from build123d import *

# Parameters (mm, degrees)
SKETCH1_R           = 2.887093213
BOSS_EXTRUDE1_DEPTH = 2
SKETCH1_4_R         = 2.887093213
SKETCH1_4_R_2       = 1.270321014
BOSS_EXTRUDE2_DEPTH = 1
SKETCH1_6_R         = 1.616772199
BOSS_EXTRUDE5_DEPTH = 5.2
SKETCH3_R           = 5.75
SKETCH3_R_2         = 2.5
SKETCH3_R_3         = 1.1
BOSS_EXTRUDE6_DEPTH = 2.5


with BuildPart() as part:
    # Sketch1 → Boss-Extrude1 (new body)
    with BuildSketch(Plane(origin=(0, 0, 0), x_dir=(1, 0, 0), z_dir=(0, 1, 0))):
        with BuildLine():
            ThreePointArc((45.240075768, -14.546907598), (42.468466284, -11.775298114), (39.6968568, -14.546907598))
            Line((39.6968568, -14.546907598), (35.935854194, -35.366456871))
            ThreePointArc((35.935854194, -35.366456871), (42.66543851, -43.184357012), (48.924361083, -34.984798737))
            Line((48.924361083, -34.984798737), (45.240075768, -14.546907598))
        make_face()
        with Locations(Location((42.470401728, -36.546907513, 0), (0, 0, 270))):
            Circle(SKETCH1_R, mode=Mode.SUBTRACT)
    extrude(amount=BOSS_EXTRUDE1_DEPTH)

    # Sketch1_4 → Boss-Extrude2 (add)
    with BuildSketch(Plane(origin=(0, 0, 0), x_dir=(1, 0, 0), z_dir=(0, 1, 0))):
        with Locations(Location((42.470401728, -36.546907513, 0), (0, 0, 270))):
            Circle(SKETCH1_4_R)
        with Locations(Location((42.470401728, -36.546907513, 0), (0, 0, 270))):
            Circle(SKETCH1_4_R_2, mode=Mode.SUBTRACT)
    extrude(amount=BOSS_EXTRUDE2_DEPTH)

    # Sketch1_6 → Boss-Extrude5 (add)
    with BuildSketch(Plane(origin=(0, 0, 0), x_dir=(1, 0, 0), z_dir=(0, 1, 0))):
        with Locations(Location((42.468466284, -14.546907598, 0), (0, 0, 270))):
            Circle(SKETCH1_6_R)
    extrude(amount=-BOSS_EXTRUDE5_DEPTH)

    # Sketch3 → Boss-Extrude6 (add)
    # profile 1 of 2: a face of its own
    with BuildSketch(Plane.XZ):
        with Locations(Location((42.470401728, 36.546907513, 0), (0, 0, 90))):
            Circle(SKETCH3_R)
        with Locations(Location((42.470401728, 36.546907513, 0), (0, 0, 270))):
            Circle(SKETCH3_R_2, mode=Mode.SUBTRACT)
    # profile 2 of 2: a face of its own
    with BuildSketch(Plane.XZ):
        with Locations((42.470401728, 36.546907513)):
            Circle(SKETCH3_R_3)
    extrude(amount=BOSS_EXTRUDE6_DEPTH)


with BuildPart() as boss_extrude6_kept_piece:
    # of the separate pieces the step leaves, the one the design keeps (boss_extrude6_pieces_kept)
    add(part.part.solids().sort_by_distance((48.924361083, 0, 34.984798737))[0])


solid = boss_extrude6_kept_piece.part
Geometry: final body of the model. Coordinates: model frame, mm. A direction names the side the tool comes from. Coordinates: 2 decimals unless noted, no trailing zeros. Loops run counter-clockwise (first coordinate to the right, second up) from the corner with the lowest first, then second, coordinate; pieces in that order, holes last. Notation, with made-up numbers: (65.5, -4) - (84.5, -4) arc R26 cw to (84.5, 21) - close; hole circle Ø10 at (56.5, 45.25). An arc over 180 degrees is marked (long way). Put each result on its own line as item: value. Start each with the question number.
Q1. Set-up query: faces 4 (the cylindrical face through (42.85, 0.49, 37.76)), 5 (the cylindrical face through (40.89, -2.56, 14.2)), 6 (the cylindrical face through (42.597, 1.493, 33.663)), 7 (the flat face through (44, -2.5, 39)). Return all of +Z, -Z, +X, -X, +Y, -Y with unobstructed straight access to the full face (end or side cutting, diameter ignored); none if empty.
Q2. Pull-direction query (Z, two-part tool) for faces 1 (the flat face through (42, -5.2, 15)), 2 (the flat face through (43, 0, 27)), 3 (the flat face through (37.843, 0.986, 24.811)); classes: released by +Z, released by -Z, zero draft, split by the parting line, or undercut.
Q3. Cut plane C-C, the plane z = 23. Return loops of the section in (x, y), and give its area (3 significant figures).
Q4. Pin query (flat end, axial travel): pin 1 Ø4 at (x, z) = (42, 36) entering from -Y; pin 2 Ø5 at (x, z) = (39.5, 17.5) entering from -Y; pin 3 Ø3 at (y, z) = (0.5, 25) entering from -X; pin 4 Ø4 at (y, z) = (-3.5, 28) entering from -X. Return the tip coordinate at first contact, or that it passes through.
Q5. Line query: line 1 (Z direction, x = 42.5, y = 0.5); line 2 (Z direction, x = 42.25, y = -0.5); line 3 (Y direction, x = 48, z = 40). Output: solid intervals per line, ascending.
Q6. Cut plane A-A, the plane x = 46.75. Return loops of the section in (y, z).
Q7. Cut plane B-B, the plane y = -1.25. Return loops of the section in (x, z).
Q8. Cut plane D-D, the plane y = 1.5. Return loops of the section in (x, z), and give its area (3 significant figures).
Filled sheet:
1. face 4: +Y, -Y
1. face 5: -Y
1. face 6: +Y
1. face 7: +Z, +X, -X, -Y
2. face 1: zero draft
2. face 2: undercut
2. face 3: released by -Z
3. outline: (38.17, 0) - (46.76, 0) - (46.76, 2) - (38.17, 2) - close
3. area: 17.2 mm²
4. pin 1: y = -2.5
4. pin 2: y = 0
4. pin 3: x = 37.54
4. pin 4: through
5. line 1: 11.78 to 35.28, 37.82 to 43.19
5. line 2: 12.94 to 16.15, 30.8 to 34.06, 39.04 to 42.29
5. line 3: 0 to 2
6. outline: (-2.5, 32.71) - (0, 32.71) - (0, 22.92) - (2, 22.92) - (2, 41.62) - (0, 41.62) - (0, 40.39) - (-2.5, 40.39) - close
7. outline: circle Ø11.5 at (42.47, 36.55); circle Ø3.23 at (42.47, 14.55); hole circle Ø5 at (42.47, 36.55)
8. outline: (35.94, 35.37) - (39.7, 14.55) arc R2.77 ccw to (45.24, 14.55) - (48.92, 34.98) arc R6.64 ccw (long way) to start; hole circle Ø5.77 at (42.47, 36.55)
8. area: 264 mm²
